Study the drawing (mm; zero at the part's minimum x, y, z) and answer. A direction names the side the tool comes from. Round coordinates to 2 decimals unless told otherwise and drop trailing zeros. Order: outer loops, then holes, each group sorted by start corner. A loop starts at its lowest first (then second) coordinate and runs counter-clockwise, first axis right, second up. Notation, with made-up numbers: M 79.5,-4 L 134.5,-4 A13 ccw 134.5,0 Z; hole C 14.25,75 d2. An arc over 180 degrees is marked long. Put each result on its own line as item: value. Start each with the question number.
1. The part is cut by section D-D (z = 4.5). Give the vertices of the cut face in (x, y).
2. The mould has two halves that part along Y. Classify the marked faces 3, 4, 5 and 6: +Y half, -Y half, draft (parallel to the pull), parting line (faces both ways), or undercut.
3. Each of these flat-tipped pins is pushed along its axis until it touches: pin 1 Ø1 at (x, y) = (1, 1) entering from -Z; pin 2 Ø1 at (y, z) = (4, 6.5) entering from +X; pin 3 Ø1.5 at (x, z) = (1.5, 4) entering from +Y. Where does it stop, or does it pass through?
4. Consider line 1 (Z direction, x = 4.5, y = 4.25); line 2 (Z direction, x = 2.75, y = 0.75); line 3 (X direction, y = 3.75, z = 5.5). Determine where each line is inside the solid, lowest interval first.
5. The part is cut by section B-B (x = 3). Give the vertices of the cut face in (y, z), then the cut area to 3 significant figures.
6. Which of the six approach directions +Z, -Z, +X, -X, +Y, -Y give full straight-line access (tool end or side, diameter ignored) to the marked faces 1 and 2?
7. The part is cut by section C-C (y = 3.55). Give the vertices of the cut face in (x, z), then the cut area to 3 significant figures.
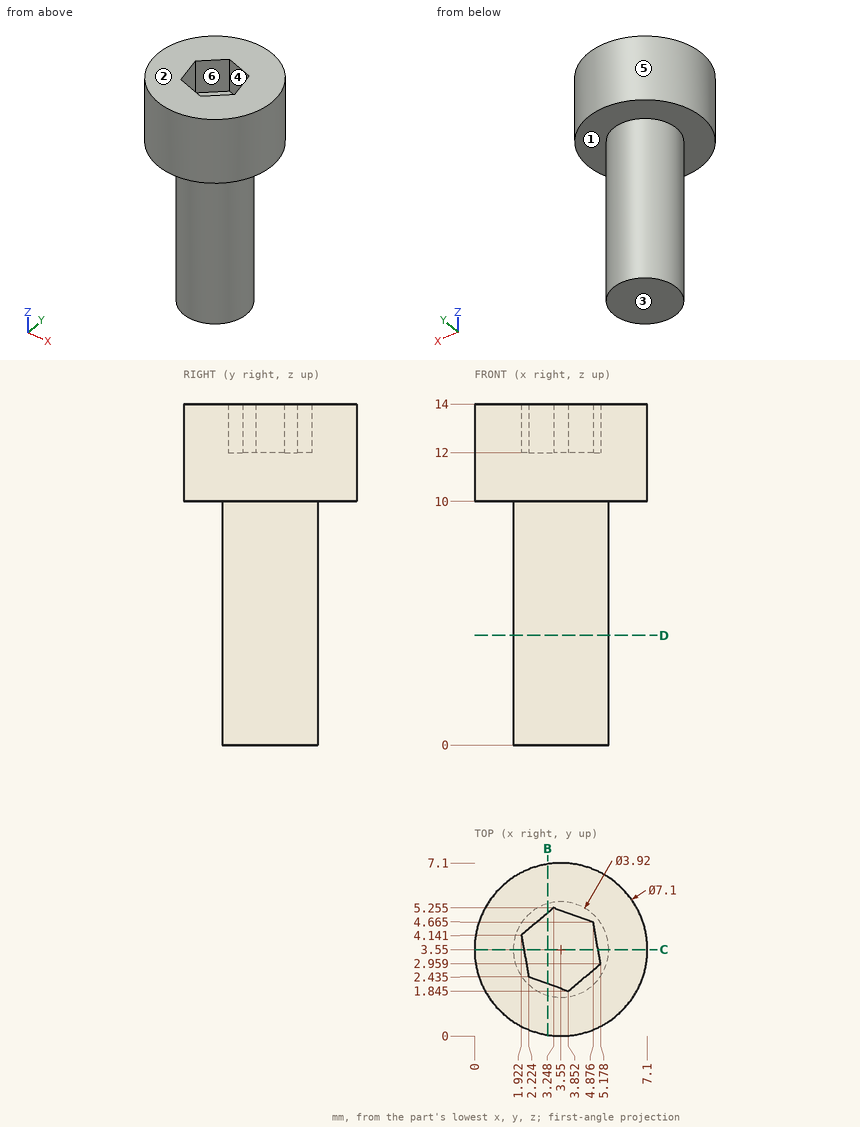
Resolved:
1. outline: C 3.55,3.55 d3.92
2. face 3: draft
2. face 4: undercut
2. face 5: parting line
2. face 6: undercut
3. pin 1: z = 10
3. pin 2: x = 5.51
3. pin 3: y = 5.02
4. line 1: 0 to 12
4. line 2: 10 to 14
4. line 3: 1.6 to 5.5
5. outline: M 0.04,10 L 1.67,10 L 1.67,0 L 5.43,0 L 5.43,10 L 7.06,10 L 7.06,14 L 5.05,14 L 5.05,12 L 2.15,12 L 2.15,14 L 0.04,14 Z
5. area: 59.9 mm2
6. face 1: -Z
6. face 2: +Z, +X, -X, +Y, -Y
7. outline: M 0,10 L 1.59,10 L 1.59,0 L 5.51,0 L 5.51,10 L 7.1,10 L 7.1,14 L 5.07,14 L 5.07,12 L 2.03,12 L 2.03,14 L 0,14 Z
7. area: 61.5 mm2
